Model file for the job. Use its own axes, mm. Round coordinates to 2 decimals unless told otherwise and drop trailing zeros. Write each loop counter-clockwise with the first axis right and the second up, starting at its lowest first coordinate (ties: lowest second). Pieces come first, ordered by that corner, then holes.
```python
from build123d import *

# Parameters (mm, degrees)
F0_W     = 2000
F0_H     = 1000
F1_DEPTH = 60
F3_DEPTH = 50
F5_DEPTH = 30


with BuildPart() as f1:
    # F0 (on Front) → F1 (new body)
    with BuildSketch(Plane.XZ):
        with Locations((0.223722, 171.635427)):
            Rectangle(F0_W, F0_H)
    extrude(amount=F1_DEPTH)

    # F2 (on face) → F3 (cut)
    with BuildSketch(Plane.XZ.offset(60)):
        with BuildLine():
            Line((66.574438, 432.670482), (-633.425562, 432.670482))
            ThreePointArc((-633.425562, 432.670482), (-783.425562, 282.670482), (-633.425562, 132.670482))
            Line((-633.425562, 132.670482), (66.574438, 132.670482))
            ThreePointArc((66.574438, 132.670482), (216.574438, 282.670482), (66.574438, 432.670482))
        make_face()
        with BuildLine():
            ThreePointArc((-633.425562, 172.670482), (-743.425562, 282.670482), (-633.425562, 392.670482))
            Line((-633.425562, 392.670482), (66.574438, 392.670482))
            ThreePointArc((66.574438, 392.670482), (176.574438, 282.670482), (66.574438, 172.670482))
            Line((66.574438, 172.670482), (-633.425562, 172.670482))
        make_face(mode=Mode.SUBTRACT)
    extrude(amount=-F3_DEPTH, mode=Mode.SUBTRACT)

    # F4 (on face) → F5 (cut)
    with BuildSketch(Plane.XZ.offset(60)):
        with BuildLine():
            Line((518.270671, 447.670482), (-463.444501, 447.670482))
            ThreePointArc((-463.444501, 447.670482), (-628.444501, 282.670482), (-463.444501, 117.670482))
            Line((-463.444501, 117.670482), (518.270671, 117.670482))
            ThreePointArc((518.270671, 117.670482), (683.270671, 282.670482), (518.270671, 447.670482))
        make_face()
        with BuildLine():
            ThreePointArc((-463.444501, 188.270956), (-558.16412, 282.990575), (-463.444501, 377.710193))
            Line((-463.444501, 377.710193), (518.270671, 377.710193))
            ThreePointArc((518.270671, 377.710193), (612.99029, 282.990575), (518.270671, 188.270956))
            Line((518.270671, 188.270956), (-463.444501, 188.270956))
        make_face(mode=Mode.SUBTRACT)
    extrude(amount=-F5_DEPTH, mode=Mode.SUBTRACT)


solid = f1.part
```
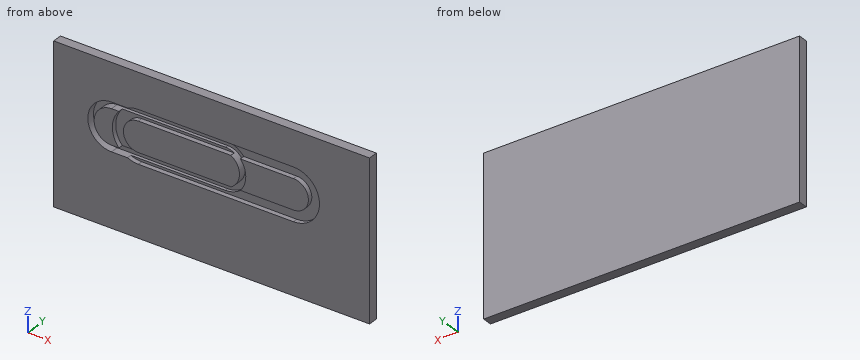
1) Cut at B-B on x = -222. List the corners of the cut face in (y, z), and give its area (3 significant figures).
2) Wall check: probe 1 along Z at (x, y) = (448.5, -53.5); probe 2 along Z at (x, y) = (-634, -30.5); probe 3 along X at (y, z) = (-43.5, 261). Give the ranges that are in metal, low to high.
3) Cut at A-A on y = -40.5. List the corners of the cut face in (x, z), and give its area (3 significant figures).
4) Cut at D-D on x = -653.5. List the corners of the cut face in (y, z).
5) Cut at C-C on z = 313. List the corners of the cut face in (x, y).
Result sheet:
1. outline: (-60, -328.36) - (0, -328.36) - (0, 671.64) - (-60, 671.64) - (-60, 447.67) - (-30, 447.67) - (-30, 432.67) - (-10, 432.67) - (-10, 392.67) - (-30, 392.67) - (-30, 377.71) - (-60, 377.71) - (-60, 188.27) - (-30, 188.27) - (-30, 172.67) - (-10, 172.67) - (-10, 132.67) - (-30, 132.67) - (-30, 117.67) - (-60, 117.67) - close
1. area: 54,200 mm2
2. probe 1: z = -328.36 to 117.67, 188.27 to 377.71, 447.67 to 671.64
2. probe 2: z = -328.36 to 132.67, 172.67 to 392.67, 432.67 to 671.64
2. probe 3: x = -999.78 to -781.85, -741.27 to -627.02, -555.58 to 174.42, 215 to 610.4, 681.84 to 1000.22
3. outline: (-999.78, -328.36) - (1000.22, -328.36) - (1000.22, 671.64) - (-999.78, 671.64) - close; (-633.43, 172.67) - (-586.43, 172.67) arc R165 cw to (-586.43, 392.67) - (-633.43, 392.67) arc R110 ccw to start; (-463.44, 188.27) - (123.04, 188.27) arc R110 ccw to (121.96, 377.71) - (-463.44, 377.71) arc R94.72 ccw to start; (182.62, 377.71) arc R150 cw to (183.15, 188.27) - (518.27, 188.27) arc R94.72 ccw to (518.27, 377.71) - close; hole (-633.43, 132.67) - (-532.18, 132.67) arc R165 ccw to (-463.44, 117.67) - (518.27, 117.67) arc R165 ccw to (518.27, 447.67) - (-463.44, 447.67) arc R165 ccw to (-532.18, 432.67) - (-633.43, 432.67) arc R150 ccw to start
3. area: 1,770,000 mm2
4. outline: (-60, -328.36) - (0, -328.36) - (0, 671.64) - (-60, 671.64) - (-60, 431.32) - (-10, 431.32) - (-10, 390.82) - (-60, 390.82) - (-60, 174.52) - (-10, 174.52) - (-10, 134.02) - (-60, 134.02) - close
5. outline: (-999.78, -60) - (-780.33, -60) - (-780.33, -10) - (-739.16, -10) - (-739.16, -60) - (-625.63, -60) - (-625.63, -30) - (-553.28, -30) - (-553.28, -60) - (172.31, -60) - (172.31, -10) - (213.48, -10) - (213.48, -60) - (608.11, -60) - (608.11, -30) - (680.46, -30) - (680.46, -60) - (1000.22, -60) - (1000.22, 0) - (-999.78, 0) - close
